Here's how the part is built. I have some questions about the finished solid (model axes, mm). Round coordinates to 2 decimals unless told otherwise and drop trailing zeros. Order: outer loops, then holes, each group sorted by start corner. A loop starts at its lowest first (then second) coordinate and runs counter-clockwise, first axis right, second up. Notation, with made-up numbers: (45.5, -2) -> (72.5, -2) arc R18 cw to (72.5, 29) -> close; hole circle Ø7 at (54, -8). An arc over 180 degrees is marked (long way). One line per item, written item: value.
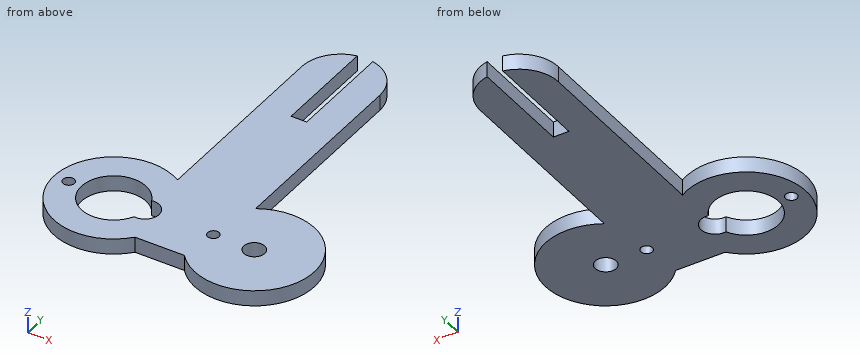
```python
from build123d import *

# Parameters (mm, degrees)
SKETCH3_R           = 1.1
BOSS_EXTRUDE1_DEPTH = 3
SKETCH5_R           = 2
CUT_EXTRUDE1_DEPTH  = 3


with BuildPart() as part:
    # Sketch3 → Boss-Extrude1 (new body)
    with BuildSketch(Plane.XY):
        with BuildLine():
            ThreePointArc((21.010133, 56.127810971), (3.63133679, 44.514906989), (23.766391, 38.905835))
            Line((23.766391, 38.905835), (33.206061, 38.905835))
            Line((33.206061, 38.905835), (33.264681316, 38.905835))
            ThreePointArc((33.264681316, 38.905835), (53.399016999, 44.544189703), (36.010134, 56.154928922))
            Line((36.010134, 56.154928922), (36.010134, 56.158016))
            Line((36.010134, 56.158016), (36.010134, 93.713691502))
            ThreePointArc((36.010134, 93.713691502), (34.319609023, 98.457108027), (30.010134, 101.062160821))
            Line((30.010134, 101.062160821), (30.010134, 101.052906355))
            Line((30.010134, 101.052906355), (30.010134, 81.052906536))
            Line((30.010134, 81.052906536), (27.010134, 81.052906536))
            Line((27.010134, 81.052906536), (27.010134, 101.052906536))
            Line((27.010134, 101.052906536), (27.010134, 101.062160866))
            ThreePointArc((27.010134, 101.062160866), (22.700658897, 98.4571082), (21.010133, 93.713692))
            Line((21.010133, 93.713692), (21.010133, 56.128782))
            Line((21.010133, 56.128782), (21.010133, 56.127810971))
        make_face()
        with Locations((6.326226, 46.332725)):
            Circle(SKETCH3_R, mode=Mode.SUBTRACT)
        with BuildLine():
            ThreePointArc((20.582059495, 43.663146925), (8.78622584, 46.332725409), (20.582059481, 49.002303953))
            ThreePointArc((20.582059481, 49.002303953), (23.686226, 46.332725447), (20.582059495, 43.663146925))
        make_face(mode=Mode.SUBTRACT)
        with Locations((34.126226, 46.332725)):
            Circle(SKETCH3_R, mode=Mode.SUBTRACT)
    extrude(amount=BOSS_EXTRUDE1_DEPTH)

    # Sketch5 → Cut-Extrude1 (cut)
    with BuildSketch(Plane.XY.offset(3)):
        with Locations((41.986225603, 46.332725741)):
            Circle(SKETCH5_R)
    extrude(amount=-CUT_EXTRUDE1_DEPTH, mode=Mode.SUBTRACT)


solid = part.part
```
Q1. I want a section at C-C on z = 0.7. Write out the boundary of the cut face in (x, y), then the cut area to 3 significant figures.
Answers:
outline: (21.01, 56.13) arc R11.5 ccw (long way) to (23.77, 38.91) -> (33.26, 38.91) arc R11.51 ccw (long way) to (36.01, 56.15) -> (36.01, 93.71) arc R7.5 ccw to (30.01, 101.06) -> (30.01, 81.05) -> (27.01, 81.05) -> (27.01, 101.06) arc R7.5 ccw to (21.01, 93.71) -> close; hole circle Ø2.2 at (6.33, 46.33); hole (20.58, 43.66) arc R2.7 ccw (long way) to (20.58, 49) arc R6.2 ccw (long way) to start; hole circle Ø2.2 at (34.13, 46.33); hole circle Ø4 at (41.99, 46.33)
area: 1,380 mm2
Q2. I want a section at D-D on y = 78.5. Write out the boundary of the cut face in (x, z).
Answers:
outline: (21.01, 0) -> (36.01, 0) -> (36.01, 3) -> (21.01, 3) -> close
Q3. I want a section at A-A on y = 87. Write out the boundary of the cut face in (x, z), then the cut area to 3 significant figures.
Answers:
outline: (21.01, 0) -> (27.01, 0) -> (27.01, 3) -> (21.01, 3) -> close; (30.01, 0) -> (36.01, 0) -> (36.01, 3) -> (30.01, 3) -> close
area: 36.0 mm2
Q4. I want a section at B-B on x = 13.5. Write out the boundary of the cut face in (y, z), then the cut area to 3 significant figures.
Answers:
outline: (34.93, 0) -> (40.31, 0) -> (40.31, 3) -> (34.93, 3) -> close; (52.35, 0) -> (57.74, 0) -> (57.74, 3) -> (52.35, 3) -> close
area: 32.3 mm2
Q5. I need wall thicknesses on line 1 along X through (y, z) = (84, 2.3); line 2 along X through (y, z) = (45.5, 1.8); line 3 along X through (y, z) = (56.5, 2.2). Which ranges of each line are inside material? Lowest first, please.
Answers:
line 1: 21.01 to 27.01, 30.01 to 36.01
line 2: 3.52 to 5.61, 7.04 to 8.84, 23.55 to 33.41, 34.84 to 40.17, 43.8 to 53.51
line 3: 9.61 to 20.36, 21.01 to 36.01, 36.61 to 47.46
Q6. For P1, Ø1.5, axis at x = 29, z = 2, coming from the +Y side; P2, Ø0.9, axis at y = 68, z = 1.5, coming from the -X side; P3, Ø0.9, axis at x = 30.5, z = 1, coming from the -Y side, each with a flat end and sliding along its axis, tell me the tip position at first contact or that it passes through.
Answers:
P1: y = 81.05
P2: x = 21.01
P3: y = 38.91
